Autodesk Inventor part; units mm, degrees
ref_plane "YZ Plane" through (0, 0, 0) normal (1, 0, 0) x (0, 1, 0)
ref_plane "XZ Plane" through (0, 0, 0) normal (0, 1, 0) x (-1, 0, 0)
ref_plane "XY Plane" through (0, 0, 0) normal (0, 0, 1) x (1, 0, 0)
sketch "Sketch1" plane through (0, 0, 0) normal (0, 0, 1) x (1, 0, 0)
  line L0 (25.85, -1.5771) -> (25.85, -14.5436) construction
  line L1 (25.85, 20.3743) -> (25.85, 33.3441) construction
  line L2 (-26.05, 20.3743) -> (-26.05, 33.3441) construction
  line L3 (-26.05, -1.5771) -> (-26.05, -14.5436) construction
  line L4 (25.85, 20.3743) -> (25.85, 33.3441) construction
  point P0 (0, 0)
ref_plane "Work Plane1" through (25.85, 33.3441, 0) normal (0, 0, 1) x (-1, 0, 0)
sketch "Sketch4" plane through (25.85, 33.3441, 0) normal (0, 0, 1) x (-1, 0, 0)
  line L0 (65.2627, -3.6865) -> (0, -3.6865) construction
  line L1 (55.9, 41.8613) -> (55.9, -3.6865) construction
  line L2 (55.9, -3.6865) -> (0, -3.6865) construction
  line L3 (0, 34.4434) -> (51.9, 0.3135) construction
  line L4 (51.9, 34.4434) -> (0, 0.3135) construction
  line L5 (50.8011, 36.1145) -> (-1.0989, 1.9846) construction
  line L6 (52.9989, 32.7724) -> (1.0989, -1.3575) construction
  line L7 (1.0989, 36.1145) -> (52.9989, 1.9846) construction
  line L8 (-1.0989, 32.7724) -> (50.8011, -1.3575) construction
  line L9 (0, 0.3135) -> (51.9, 0.3135) construction
  line L10 (51.9, 0.3135) -> (51.9, 34.4434) construction
  line L11 (51.9, 34.4434) -> (0, 34.4434) construction
  line L12 (0, 34.4434) -> (0, 0.3135) construction
  line L13 (0, 34.4434) -> (0, 29.4434) construction
  line L14 (0, 34.4434) -> (5, 34.4434) construction
  line L15 (0, 29.4434) -> (3.9633, 29.4434)
  line L16 (0, 0.3135) -> (0, 5.3135) construction
  line L17 (0, 0.3135) -> (5, 0.3135) construction
  line L18 (51.9, 0.3135) -> (51.9, 5.3135) construction
  line L19 (51.9, 0.3135) -> (56.9, 0.3135) construction
  line L20 (51.9, 34.4434) -> (51.9, 29.4434) construction
  line L21 (51.9, 34.4434) -> (56.9, 34.4434) construction
  line L22 (51.9, 29.4434) -> (47.9367, 29.4434)
  line L23 (3.9633, 5.3135) -> (22.31, 17.3785)
  line L24 (47.9367, 5.3135) -> (29.59, 17.3785)
  line L25 (47.9367, 29.4434) -> (29.59, 17.3785)
  line L26 (3.64, 34.4434) -> (25.95, 19.7722)
  line L27 (25.95, 19.7722) -> (48.26, 34.4434)
  line L28 (3.64, 0.3135) -> (25.95, 14.9848)
  line L29 (48.26, 0.3135) -> (25.95, 14.9848)
  line L30 (22.31, 17.3785) -> (3.9633, 29.4434)
  line L31 (51.9, 5.3135) -> (51.9, 0.3135)
  line L32 (51.9, 29.4434) -> (51.9, 34.4434)
  line L33 (0, 5.3135) -> (3.9633, 5.3135)
  line L34 (51.9, 5.3135) -> (47.9367, 5.3135)
  line L35 (51.9, 34.4434) -> (48.26, 34.4434)
  line L36 (0, 34.4434) -> (3.64, 34.4434)
  line L37 (0, 34.4434) -> (0, 29.4434)
  line L38 (3.64, 0.3135) -> (0, 0.3135)
  line L39 (48.26, 0.3135) -> (51.9, 0.3135)
  line L40 (0, 0.3135) -> (0, 5.3135)
  point P0 (25.85, 33.3441)
  point P1 (25.95, 17.3785)
  dimension "d17" = 2
  dimension "d18" = 2
  dimension "d19" = 2
  dimension "d20" = 2
  dimension "d21" = 5
  dimension "d22" = 90
  dimension "d23" = 5
  dimension "d24" = 90
  dimension "d25" = 5
  dimension "d26" = 90
  dimension "d27" = 5
  dimension "d28" = 90
extrude "Extrusion1" add sketch "Sketch4" along normal blind 110
Here's how the part is built. I have some questions about the finished solid (model axes, mm). A direction names the side the tool comes from. Coordinates: 2 decimals unless noted, no trailing zeros. Order: outer loops, then holes, each group sorted by start corner. A loop starts at its lowest first (then second) coordinate and runs counter-clockwise, first axis right, second up. Notation, with made-up numbers: (-5, -15.75) -> (44, -15.75) arc R18 ccw to (44, 6.25) -> close; hole circle Ø3 at (76, 35.5). An arc over 180 degrees is marked (long way). Answer in a Markdown table with one row per item.
(1) On a 3-axis mill with a long thin cutter (end or side, diameter ignored), from which of +Z, -Z, +X, -X, +Y, -Y can I reach the whole of each face in a straight line? I mean faces 1 (the face through (24, 3.901, 54)), 2 (the face through (-11.411, 25.798, 54.23)), 3 (the face through (11.211, 6.134, 54.23)), 4 (the face through (-24, 28.031, 54)). Say none if no direction works.
Answer key:
| item | result |
|---|---|
| face 1 | +Z, -Z, +X |
| face 2 | +Z, -Z, +Y |
| face 3 | +Z, -Z, -Y |
| face 4 | +Z, -Z, -X |
(2) I want a section at D-D on x = 1. List the corners of the cut face in (y, z) for me.
Answer key:
| item | result |
|---|---|
| outline | (12.85, 0) -> (19.08, 0) -> (19.08, 110) -> (12.85, 110) -> close |
(3) I want a section at B-B on z = 60. List the corners of the cut face in (x, y) for me, then the cut area to 3 significant figures.
Answer key:
| item | result |
|---|---|
| outline | (-26.05, -1.1) -> (-22.41, -1.1) -> (-0.1, 13.57) -> (22.21, -1.1) -> (25.85, -1.1) -> (25.85, 3.9) -> (21.89, 3.9) -> (3.54, 15.97) -> (21.89, 28.03) -> (25.85, 28.03) -> (25.85, 33.03) -> (22.21, 33.03) -> (-0.1, 18.36) -> (-22.41, 33.03) -> (-26.05, 33.03) -> (-26.05, 28.03) -> (-22.09, 28.03) -> (-3.74, 15.97) -> (-22.09, 3.9) -> (-26.05, 3.9) -> close |
| area | 483 mm^2 |
(4) I want a section at A-A on x = 7. List the corners of the cut face in (y, z) for me.
Answer key:
| item | result |
|---|---|
| outline | (8.9, 0) -> (13.69, 0) -> (13.69, 110) -> (8.9, 110) -> close; (18.24, 0) -> (23.03, 0) -> (23.03, 110) -> (18.24, 110) -> close |
(5) Will these pins go through, and if not, where does the flat tip stop? pin 1 Ø3 at (y, z) = (27.5, 19) entering from -X; pin 2 Ø2 at (y, z) = (24.5, 38.5) entering from +X; pin 3 Ø1.5 at (x, z) = (-4.5, 44) entering from +Y; pin 4 Ø1.5 at (x, z) = (-8, 42) entering from -Y.
Answer key:
| item | result |
|---|---|
| pin 1 | x = -26.05 |
| pin 2 | x = 18.04 |
| pin 3 | y = 21.75 |
| pin 4 | y = 7.88 |
(6) I want a section at C-C on y = 10. List the corners of the cut face in (x, z) for me, then the cut area to 3 significant figures.
Answer key:
| item | result |
|---|---|
| outline | (-12.81, 0) -> (-5.53, 0) -> (-5.53, 110) -> (-12.81, 110) -> close; (5.33, 0) -> (12.61, 0) -> (12.61, 110) -> (5.33, 110) -> close |
| area | 1,600 mm^2 |
(7) Please list where these lines run through material, in increasing order: probe 1 along Y at (x, z) = (-10, 23); probe 2 along X at (y, z) = (24, 95.5); probe 3 along Y at (x, z) = (-21, 50.5).
Answer key:
| item | result |
|---|---|
| probe 1 | 7.06 to 11.85, 20.08 to 24.87 |
| probe 2 | -15.96 to -8.68, 8.48 to 15.76 |
| probe 3 | -0.17 to 4.62, 27.32 to 32.1 |
(8) Thinking about a two-plate mould opening in Y: for faces 5 (the face through (-26.05, 1, 54)), 6 (the face through (24, -1.099, 54)), 7 (the face through (-24, 3.901, 54)), 8 (the face through (11.211, 25.798, 54.23)), which applies, +Y half, -Y half, draft (parallel to the pull), parting line (faces both ways), or undercut?
Answer key:
| item | result |
|---|---|
| face 5 | draft |
| face 6 | -Y half |
| face 7 | undercut |
| face 8 | +Y half |
